from build123d import *

# Parameters (mm, degrees)
SKETCH1_R           = 1.4225
BOSS_EXTRUDE1_DEPTH = 1.5
SKETCH2_R           = 2.0225
SKETCH2_R_2         = 1.4225
BOSS_EXTRUDE2_DEPTH = 1.5
FILLET1_R           = 0.5
FILLET2_R           = 0.5


with BuildPart() as part:
    # Sketch1 → Boss-Extrude1 (new body)
    with BuildSketch(Plane(origin=(0, 0, 0), x_dir=(1, 0, 0), z_dir=(0, 1, 0))):
        Polygon((-8.25, -3.375), (-8.25, 3.375), (8.25, 3.375), (8.25, -3.375), (0.875, -3.375), (0.875, 0.125), (-0.875, 0.125), (-0.875, -3.375), align=None)
        with Locations((-5, 0)):
            Circle(SKETCH1_R, mode=Mode.SUBTRACT)
        with Locations((5, 0)):
            Circle(SKETCH1_R, mode=Mode.SUBTRACT)
    extrude(amount=BOSS_EXTRUDE1_DEPTH)

    # Sketch2 → Boss-Extrude2 (add)
    with BuildSketch(Plane.XZ):
        with Locations((5, 0)):
            Circle(SKETCH2_R)
        with Locations((5, 0)):
            Circle(SKETCH2_R_2, mode=Mode.SUBTRACT)
        with Locations((-5, 0)):
            Circle(SKETCH2_R)
        with Locations((-5, 0)):
            Circle(SKETCH2_R_2, mode=Mode.SUBTRACT)
    extrude(amount=BOSS_EXTRUDE2_DEPTH)

    # Fillet1
    fillet1_edges = [part.edges().sort_by_distance(p)[0] for p in [
        (2.9775, -1.5, 0),
        (-7.0225, -1.5, 0),
    ]]
    fillet(fillet1_edges, radius=FILLET1_R)

    # Fillet2
    fillet2_edges = [part.edges().sort_by_distance(p)[0] for p in [
        (-8.25, 1.5, 0),
        (-4.5625, 1.5, 3.375),
        (8.25, 0.75, 3.375),
        (-8.25, 0.75, 3.375),
        (-8.25, 0.75, -3.375),
        (8.25, 0.75, -3.375),
        (-0.875, 1.5, 1.625),
        (0, 1.5, -0.125),
        (0.875, 1.5, 1.625),
        (4.5625, 1.5, 3.375),
        (8.25, 1.5, 0),
        (0, 1.5, -3.375),
    ]]
    fillet(fillet2_edges, radius=FILLET2_R)


solid = part.part
The model under review builds one solid part; all positions refer to its coordinate system, in mm. A direction names the side the tool comes from. Round coordinates to 2 decimals unless told otherwise and drop trailing zeros. Loops run counter-clockwise (first coordinate to the right, second up) from the corner with the lowest first, then second, coordinate; pieces in that order, holes last. Notation, with made-up numbers: (56.25, 48.5) -> (115.25, 48.5) arc R15 ccw to (115.25, 64.5) -> close; hole circle Ø9 at (16, -9). An arc over 180 degrees is marked (long way). One line per question, with ' | ' between items. Start each with the question number.
Item 1: Draft analysis for pull direction X (two halves, no side actions). For faces 4 (the face through (-3.07, -0.49, 0.61)), 5 (the face through (8.25, 0.5, 0)), 6 (the face through (-0.1, 0.5, -3.375)), state which applies: +X half, -X half, draft (parallel to the pull), parting line (faces both ways), or undercut.
Item 2: Add section D-D, the plane x = -2.75. Write out the cut boundary in (y, z) (3 decimals).
Item 3: Add section C-C, the plane y = 1.15. Count the separate pieces of the cut face and the enclosed holes in it, then the cut area to 3 significant figures.
Item 4: For pin 1 (1 mm diameter, centred on y = -1, z = 0.5, fed in from -X); pin 2 (1.1 mm diameter, centred on x = 0.5, y = 0.5, fed in from +Z) (3 decimals), all flat-tipped, find the tip position at first contact; note any pin that passes through.
Item 5: Add section B-B, the plane y = -0.65. Write out the cut boundary in (x, z) (1 decimal).
Item 6: Machinability: for faces 1 (the face through (0, 0, -1)), 2 (the face through (0, 1.5, -1)), 3 (the face through (0, 0.5, -0.125)), which of the approach directions +Z, -Z, +X, -X, +Y, -Y give a long, thin tool a straight path to every point of the face, cutting with its end or side? Answer none if there is none.
Item 7: Wall thickness on line 1 along Z through (x, y) = (5, -0.1); line 2 along Z through (x, y) = (-5, 0.4) (1 decimal); line 3 along X through (y, z) = (0.7, 0.25) (3 decimals): over which ranges is each line inside the solid? List them lowest first. Write a range as [from, to].
Return value:
1) face 4: undercut | face 5: +X half | face 6: draft
2) outline: (0, -3.375) -> (1, -3.375) arc R0.5 ccw to (1.5, -2.875) -> (1.5, 2.875) arc R0.5 ccw to (1, 3.375) -> (0, 3.375) -> close
3) separate pieces: 1 | enclosed holes: 2 | area: 91.1 mm2
4) pin 1: stops at x = -7.02 | pin 2: stops at z = 3.375
5) outline: circle Ø4 at (-5, 0); circle Ø4 at (5, 0); hole circle Ø2.8 at (-5, 0); hole circle Ø2.8 at (5, 0)
6) face 1: -Y | face 2: +Z, -Z, +X, -X, +Y | face 3: +Z, +Y, -Y
7) line 1: z = [-2.02, -1.42], [1.42, 2.02] | line 2: z = [-3.4, -1.4], [1.4, 3.4] | line 3: x = [-8.25, -6.4], [-3.6, -0.875], [0.875, 3.6], [6.4, 8.25]
